For this review, take the finished solid that the model builds, in its own axes (mm). A direction names the side the tool comes from. Give positions to 0.01 mm unless a question says otherwise; leave off trailing zeros. Write each loop counter-clockwise with the first axis right and the second up, starting at its lowest first coordinate (ties: lowest second). Pieces come first, ordered by that corner, then holes. Notation, with made-up numbers: M 82,77 L 101,77 A6 ccw 101,86 Z; hole C 60,19 d4. An arc over 180 degrees is marked long. Write item = value, one per line.
```python
from build123d import *

# Parameters (mm, degrees)
SKETCH1_W           = 177.8
SKETCH1_H           = 222.25
BOSS_EXTRUDE1_DEPTH = 3.175
CUT_EXTRUDE1_DEPTH  = 240.391631276


with BuildPart() as part:
    # Sketch1 → Boss-Extrude1 (new body)
    with BuildSketch(Plane.XY):
        with Locations((0, 111.125)):
            Rectangle(SKETCH1_W, SKETCH1_H)
    extrude(amount=BOSS_EXTRUDE1_DEPTH)

    # Sketch2 → Cut-Extrude1 (cut, through all)
    with BuildSketch(Plane.XY.offset(3.175)):
        with BuildLine():
            Line((53.975, 22.225), (-53.975, 22.225))
            ThreePointArc((-53.975, 22.225), (-60.710192091, 25.014807909), (-63.5, 31.75))
            Line((-63.5, 31.75), (-63.5, 190.5))
            ThreePointArc((-63.5, 190.5), (-60.710192091, 197.235192091), (-53.975, 200.025))
            Line((-53.975, 200.025), (53.975, 200.025))
            ThreePointArc((53.975, 200.025), (60.710192091, 197.235192091), (63.5, 190.5))
            Line((63.5, 190.5), (63.5, 31.75))
            ThreePointArc((63.5, 31.75), (60.710192091, 25.014807909), (53.975, 22.225))
        make_face()
    extrude(amount=-CUT_EXTRUDE1_DEPTH, mode=Mode.SUBTRACT)


solid = part.part
```
1. Machinability: for faces 1 (the face through (78, 113, 3.175)), 2 (the face through (-60.784, 197.161, 1.61)), which of the approach directions +Z, -Z, +X, -X, +Y, -Y give a long, thin tool a straight path to every point of the face, cutting with its end or side? Answer none if there is none.
Responses:
face_1 = +Z, +X, -X, +Y, -Y
face_2 = +Z, -Z
2. The part is to be moulded in two halves that separate along X. For faces 3 (the face through (60.784, 25.089, 1.61)), 4 (the face through (78, 113, 0)), say which applies: +X half, -X half, draft (parallel to the pull), parting line (faces both ways), or undercut.
Responses:
face_3 = undercut
face_4 = draft
3. For line 1 along X through (y, z) = (106, 1.35); line 2 along Y through (x, z) = (-40, 2.25) (3 decimals); line 3 along Y through (x, z) = (-60, 1.4), list the stretches that pass through material, from the lowest coordinate up. Write a range as from..to.
Responses:
line_1 = -88.9..-63.5, 63.5..88.9
line_2 = 0..22.225, 200.025..222.25
line_3 = 0..24.37, 197.88..222.25
4. Insertion check: P1, Ø6, axis at x = -51.5, y = 27, coming from the -Z side. The pin has a flat end and moves straight along its axis. Give the tip position at first contact, or say it passes through.
Responses:
P1 = through
5. We need section C-C, the plane z = 0.8. Write out the cut boundary in (x, y) (3 decimals).
Responses:
outline = M -88.9,0 L 88.9,0 L 88.9,222.25 L -88.9,222.25 Z; hole M -63.5,31.75 A9.525 ccw -53.975,22.225 L 53.975,22.225 A9.525 ccw 63.5,31.75 L 63.5,190.5 A9.525 ccw 53.975,200.025 L -53.975,200.025 A9.525 ccw -63.5,190.5 Z
6. We need section B-B, the plane x = -45. Write out the cut boundary in (y, z) (3 decimals).
Responses:
outline = M 0,0 L 22.225,0 L 22.225,3.175 L 0,3.175 Z; M 200.025,0 L 222.25,0 L 222.25,3.175 L 200.025,3.175 Z
7. We need section A-A, the plane y = 91.5. Write out the cut boundary in (x, z) (3 decimals).
Responses:
outline = M -88.9,0 L -63.5,0 L -63.5,3.175 L -88.9,3.175 Z; M 63.5,0 L 88.9,0 L 88.9,3.175 L 63.5,3.175 Z
